Study the drawing (mm; zero at the part's minimum x, y, z) and answer. Round coordinates to 2 decimals unless told otherwise and drop trailing zeros. Loops run counter-clockwise (first coordinate to the right, second up) from the corner with the lowest first, then second, coordinate; pieces in that order, holes last. Notation, with made-up numbers: (20.25, -28) - (72.25, -28) arc R8 ccw to (72.25, -21) - close; hole circle Ø1 at (-12.75, 79). An arc over 180 degrees is marked (long way). One line per item, written item: value.
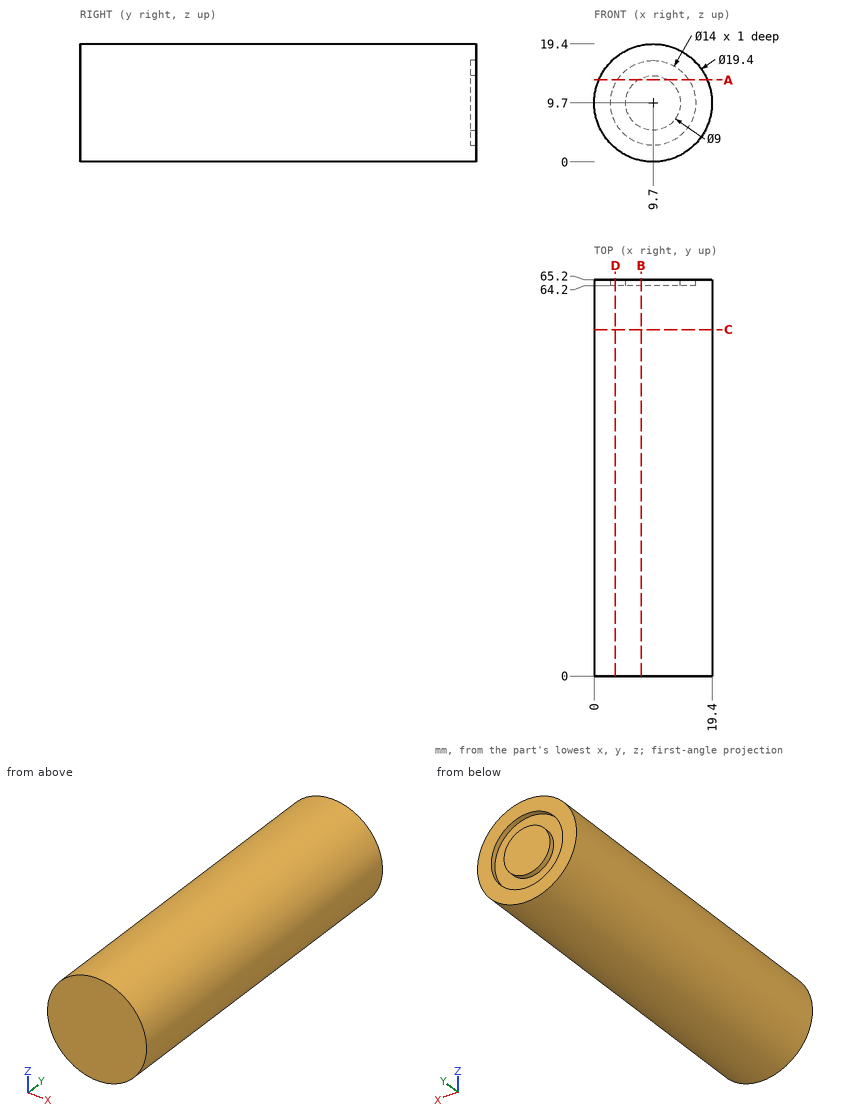
1) A cutting plane is placed at D-D on x = 3.5. Give the vertices of the cut face in (y, z).
Final values:
outline: (0, 2.24) - (65.2, 2.24) - (65.2, 6.45) - (64.2, 6.45) - (64.2, 12.95) - (65.2, 12.95) - (65.2, 17.16) - (0, 17.16) - close
2) A cutting plane is placed at A-A on z = 13.5. Give the vertices of the cut face in (x, y).
Final values:
outline: (0.78, 0) - (18.62, 0) - (18.62, 65.2) - (15.58, 65.2) - (15.58, 64.2) - (12.11, 64.2) - (12.11, 65.2) - (7.29, 65.2) - (7.29, 64.2) - (3.82, 64.2) - (3.82, 65.2) - (0.78, 65.2) - close
3) A cutting plane is placed at C-C on y = 57. Give the vertices of the cut face in (x, z).
Final values:
outline: circle Ø19.4 at (9.7, 9.7)
4) A cutting plane is placed at B-B on x = 7.75. Give the vertices of the cut face in (y, z).
Final values:
outline: (0, 0.2) - (65.2, 0.2) - (65.2, 2.98) - (64.2, 2.98) - (64.2, 5.64) - (65.2, 5.64) - (65.2, 13.76) - (64.2, 13.76) - (64.2, 16.42) - (65.2, 16.42) - (65.2, 19.2) - (0, 19.2) - close
5) Consider L1, parallel to X at y = 64.4, z = 9.7; L2, parallel to Y at x = 13.75, z = 14; L3, parallel to X at y = 33.5, z = 9.5. Determine where each line is inside the solid, lowest interval first.
Final values:
L1: 0 to 2.7, 5.2 to 14.2, 16.7 to 19.4
L2: 0 to 64.2
L3: 0 to 19.4
6) Each of these flat-tipped pins is pushed along its axis until it touches: pin 1 Ø2 at (x, y) = (14, 35.5) entering from -Z; pin 2 Ø3 at (x, y) = (3, 16) entering from -Z; pin 3 Ø3 at (y, z) = (19.5, 2.5) entering from -X; pin 4 Ø2 at (x, z) = (13.5, 15.5) entering from -Y. Where does it stop, or does it pass through?
Final values:
pin 1: z = 0.58
pin 2: z = 1.51
pin 3: x = 1.85
pin 4: y = 0
